Part model, mm, in its own coordinate system. A direction names the side the tool comes from. Give positions to 0.01 mm unless a question says otherwise; leave off trailing zeros. Loops run counter-clockwise (first coordinate to the right, second up) from the corner with the lowest first, then second, coordinate; pieces in that order, holes last. Notation, with made-up numbers: M 86,42 L 134,42 A31 cw 134,69 Z; hole C 4,89 d9. An arc over 180 degrees is marked long. Answer in a Markdown table with one row per item.
from build123d import *

# Parameters (mm, degrees)
IZIM1_W                     = 215
IZIM1_H                     = 160.7
Y_KSEKLIK_EKSTR_ZYON1_DEPTH = 9.5
IZIM2_W                     = 196.3
IZIM2_H                     = 142.3
Y_KSEKLIK_EKSTR_ZYON2_DEPTH = 27.24
IZIM3_W                     = 10
IZIM3_H                     = 26.5
IZIM3_W_2                   = 9
IZIM3_H_2                   = 25.5
KES_EKSTR_ZYON1_DEPTH       = 15
IZIM4_W                     = 9
IZIM4_H                     = 25.5
KES_EKSTR_ZYON2_DEPTH       = 5
IZIM5_R                     = 0.5
KES_EKSTR_ZYON3_DEPTH       = 5
M3_DI_LI_DELIK1_D           = 2.5
M3_DI_LI_DELIK1_DEPTH       = 8.5
M3_DI_LI_DELIK1_TIP         = 0.751075774
IZIM8_W                     = 155
IZIM8_H                     = 86
KES_EKSTR_ZYON4_DEPTH       = 0.05
KES_EKSTR_ZYON5_DEPTH       = 0.005
RADYUS1_R                   = 3
RADYUS2_R                   = 1
IZIM10_W                    = 36
IZIM10_H                    = 40
KES_EKSTR_ZYON6_DEPTH       = 7.5
RADYUS3_R                   = 1


with BuildPart() as part:
    # Çizim1 → Yükseklik-Ekstrüzyon1 (new body)
    with BuildSketch(Plane.XY):
        Rectangle(IZIM1_W, IZIM1_H)
    extrude(amount=Y_KSEKLIK_EKSTR_ZYON1_DEPTH)

    # Çizim2 → Yükseklik-Ekstrüzyon2 (add)
    with BuildSketch(Plane.XY.offset(9.5)):
        Rectangle(IZIM2_W, IZIM2_H)
    extrude(amount=Y_KSEKLIK_EKSTR_ZYON2_DEPTH)

    # Çizim3 → Kes-Ekstrüzyon1 (cut)
    with BuildSketch(Plane.XY.offset(36.74)):
        with Locations((63.15, 24.65)):
            Rectangle(IZIM3_W, IZIM3_H)
        with Locations((63.15, 24.65)):
            Rectangle(IZIM3_W_2, IZIM3_H_2, mode=Mode.SUBTRACT)
    extrude(amount=-KES_EKSTR_ZYON1_DEPTH, mode=Mode.SUBTRACT)

    # Çizim4 → Kes-Ekstrüzyon2 (cut)
    with BuildSketch(Plane.XY.offset(36.74)):
        with Locations((63.15, 24.65)):
            Rectangle(IZIM4_W, IZIM4_H)
    extrude(amount=-KES_EKSTR_ZYON2_DEPTH, mode=Mode.SUBTRACT)

    # Çizim5 → Kes-Ekstrüzyon3 (cut)
    with BuildSketch(Plane.XY.offset(31.74)):
        with BuildLine():
            Line((59.65, 33.4), (59.65, 15.9))
            Line((59.65, 15.9), (63.65, 15.9))
            ThreePointArc((63.65, 15.9), (66.618585522, 18.466987298), (64.506956825, 21.775))
            ThreePointArc((64.506956825, 21.775), (66.65, 24.65), (64.506956825, 27.525))
            ThreePointArc((64.506956825, 27.525), (66.618585522, 30.833012702), (63.65, 33.4))
            Line((63.65, 33.4), (59.65, 33.4))
        make_face()
        with Locations((63.15, 30.4)):
            Circle(IZIM5_R, mode=Mode.SUBTRACT)
        with Locations((63.15, 18.9)):
            Circle(IZIM5_R, mode=Mode.SUBTRACT)
        with Locations((63.15, 24.65)):
            Circle(IZIM5_R, mode=Mode.SUBTRACT)
    extrude(amount=-KES_EKSTR_ZYON3_DEPTH, mode=Mode.SUBTRACT)

    # M3 Dişli Delik1
    with Locations(Plane.XY.offset(31.74)):
        with Locations((63.15, 35.4), (63.15, 13.9)):
            Hole(M3_DI_LI_DELIK1_D / 2, depth=M3_DI_LI_DELIK1_DEPTH)
            with Locations((0, 0, -(M3_DI_LI_DELIK1_DEPTH + M3_DI_LI_DELIK1_TIP / 2))):  # 118° drill point
                Cone(0, M3_DI_LI_DELIK1_D / 2, M3_DI_LI_DELIK1_TIP, mode=Mode.SUBTRACT)

    # Çizim8 → Kes-Ekstrüzyon4 (cut)
    with BuildSketch(Plane(origin=(0, 0, 0), x_dir=(-1, 0, 0), z_dir=(0, 0, -1))):
        Rectangle(IZIM8_W, IZIM8_H)
    extrude(amount=-KES_EKSTR_ZYON4_DEPTH, mode=Mode.SUBTRACT)

    # Çizim9 → Kes-Ekstrüzyon5 (cut)
    with BuildSketch(Plane(origin=(0, 0, 0), x_dir=(-1, 0, 0), z_dir=(0, 0, -1))):
        with BuildLine():
            Line((-88, 61), (88, 61))
            ThreePointArc((88, 61), (90.828427125, 59.828427125), (92, 57))
            Line((92, 57), (92, -57))
            ThreePointArc((92, -57), (90.828427125, -59.828427125), (88, -61))
            Line((88, -61), (-92, -61))
            Line((-92, -61), (-92, 57))
            ThreePointArc((-92, 57), (-90.828427125, 59.828427125), (-88, 61))
        make_face()
        with BuildLine():
            Line((-88, 60), (88, 60))
            ThreePointArc((88, 60), (90.121320344, 59.121320344), (91, 57))
            Line((91, 57), (91, -57))
            ThreePointArc((91, -57), (90.121320344, -59.121320344), (88, -60))
            Line((88, -60), (-91, -60))
            Line((-91, -60), (-91, 57))
            ThreePointArc((-91, 57), (-90.121320344, 59.121320344), (-88, 60))
        make_face(mode=Mode.SUBTRACT)
    extrude(amount=-KES_EKSTR_ZYON5_DEPTH, mode=Mode.SUBTRACT)

    # Radyus1
    radyus1_edges = [part.edges().sort_by_distance(p)[0] for p in [
        (107.5, -80.35, 4.75),
        (-107.5, -80.35, 4.75),
        (-107.5, 80.35, 4.75),
        (107.5, 80.35, 4.75),
    ]]
    fillet(radyus1_edges, radius=RADYUS1_R)

    # Radyus2
    radyus2_edges = [part.edges().sort_by_distance(p)[0] for p in [
        (107.5, 0, 0),
        (0, -80.35, 0),
        (-107.5, 0, 0),
        (0, 80.35, 0),
        (106.621320344, 79.471320344, 0),
        (-106.621320344, 79.471320344, 0),
        (-106.621320344, -79.471320344, 0),
        (106.621320344, -79.471320344, 0),
    ]]
    fillet(radyus2_edges, radius=RADYUS2_R)

    # Çizim10 → Kes-Ekstrüzyon6 (cut)
    with BuildSketch(Plane.XY.offset(36.74)):
        with Locations((53.15, -18.85)):
            Rectangle(IZIM10_W, IZIM10_H)
    extrude(amount=-KES_EKSTR_ZYON6_DEPTH, mode=Mode.SUBTRACT)

    # Radyus3
    radyus3_edges = [part.edges().sort_by_distance(p)[0] for p in [
        (98.15, -71.15, 23.12),
        (98.15, 71.15, 23.12),
        (-98.15, 71.15, 23.12),
        (-98.15, -71.15, 23.12),
    ]]
    fillet(radyus3_edges, radius=RADYUS3_R)


solid = part.part
(1) Saw through at B-B (z = 14). Write the cut outline in (x, y), plus the area to 3 significant figures.
Recorded:
| item | result |
|---|---|
| outline | M -98.15,-70.15 A1 ccw -97.15,-71.15 L 97.15,-71.15 A1 ccw 98.15,-70.15 L 98.15,70.15 A1 ccw 97.15,71.15 L -97.15,71.15 A1 ccw -98.15,70.15 Z |
| area | 27,900 mm^2 |
(2) Which spindle directions (+Z, -Z, +X, -X, +Y, -Y) get a long thin tool onto all of the face, cutting with end or side? Do faces 1 (the face through (-1, 1, 36.74)), 2 (the face through (-1, 72, 9.5)), 3 (the face through (-1, -71.15, 23)), 4 (the face through (98.15, -1, 23)). Say none if no direction does.
Recorded:
| item | result |
|---|---|
| face 1 | +Z, +X, -X, +Y, -Y |
| face 2 | +Z |
| face 3 | +Z, +X, -X, -Y |
| face 4 | +Z, +X, +Y, -Y |
(3) Pin check, flat tips, straight feed: pin 1 Ø4 at (x, y) = (63.15, 13.9) entering from -Z; pin 2 Ø8 at (y, z) = (14, 25.5) entering from +X; pin 3 Ø4 at (y, z) = (-11.5, 34.5) entering from -X. Stop position of each tip, or through.
Recorded:
| item | result |
|---|---|
| pin 1 | stops at z = 0.05 |
| pin 2 | stops at x = 98.15 |
| pin 3 | stops at x = -98.15 |
(4) Drill centre lines: line 1 along X through (y, z) = (35.4, 27.25); line 2 along Y through (x, z) = (63.15, 25); line 3 along X through (y, z) = (13, 25). Where is each one in solid material? Low to high.
Recorded:
| item | result |
|---|---|
| line 1 | x = -98.15 to 58.15, 58.65 to 61.9, 64.4 to 67.65, 68.15 to 98.15 |
| line 2 | y = -71.15 to 11.4, 11.9 to 12.65, 15.15 to 34.15, 36.65 to 37.4, 37.9 to 71.15 |
| line 3 | x = -98.15 to 58.15, 58.65 to 62.28, 64.02 to 67.65, 68.15 to 98.15 |
(5) Pull direction Y, two halves, no side cores. Call faces 5 (the face through (53, -38.85, 33)), 6 (the face through (-1, -52, 0)), 7 (the face through (-1, 80.35, 5)): +Y half, -Y half, draft (parallel to the pull), parting line (faces both ways), or undercut.
Recorded:
| item | result |
|---|---|
| face 5 | undercut |
| face 6 | draft |
| face 7 | +Y half |
(6) Saw through at A-A (x = 22.5). Write the cut outline in (y, z) (3 decimals).
Recorded:
| item | result |
|---|---|
| outline | M -80.35,1 A1 ccw -79.35,0 L -61,0 L -61,0.005 L -60,0.005 L -60,0 L -43,0 L -43,0.05 L 43,0.05 L 43,0 L 60,0 L 60,0.005 L 61,0.005 L 61,0 L 79.35,0 A1 ccw 80.35,1 L 80.35,9.5 L 71.15,9.5 L 71.15,36.74 L -71.15,36.74 L -71.15,9.5 L -80.35,9.5 Z |
